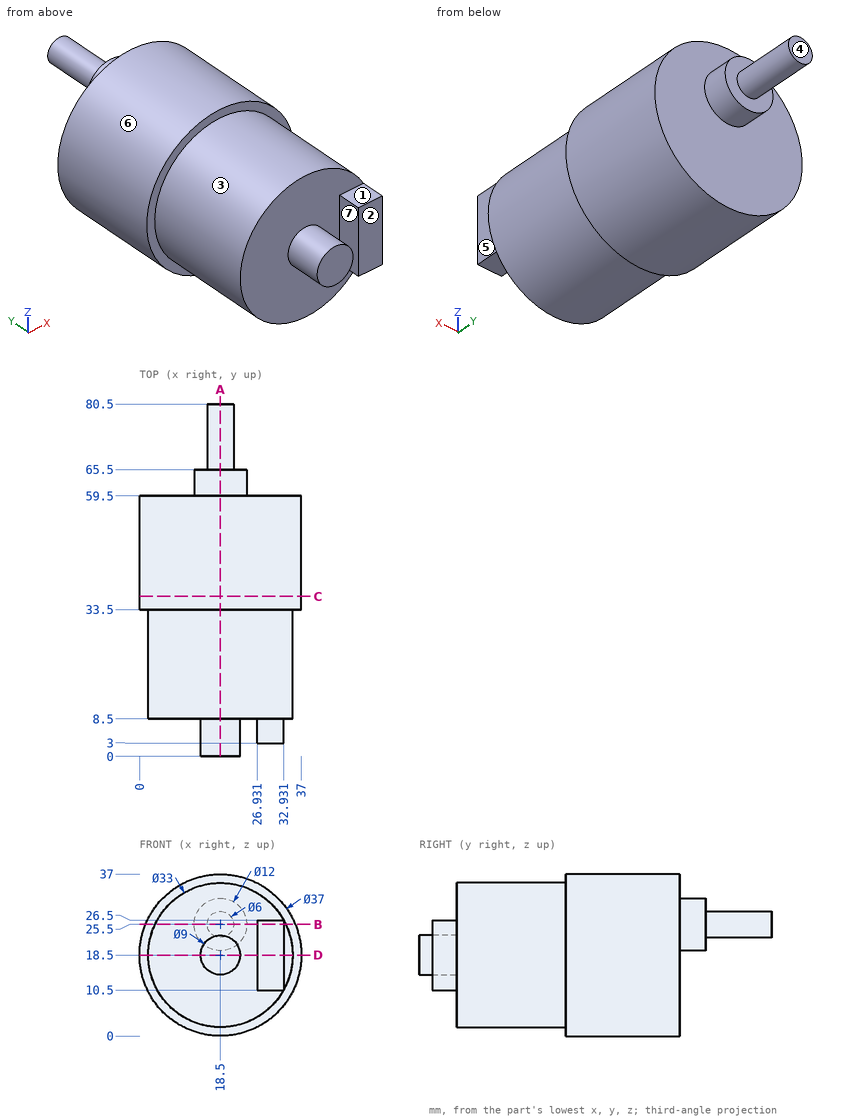
Answer from the drawing. Dimensions are ordinates in mm from the lowest x, y and z of the part. A direction names the side the tool comes from. Give positions to 0.01 mm unless a question says otherwise; leave off trailing zeros. Loops run counter-clockwise (first coordinate to the right, second up) from the corner with the lowest first, then second, coordinate; pieces in that order, holes last. Notation, with made-up numbers: (-32, -12) - (-13, -12) arc R16 ccw to (-13, 9) - close; hole circle Ø2 at (54, 81). An arc over 180 degrees is marked (long way). Write each question's results on one line, items separated by ' | '.
1. Find section D-D, the plane z = 18.5. Write down the section's boundary in (x, y), then the cut area to 3 significant figures.
Resolved:
outline: (0, 33.5) - (2, 33.5) - (2, 8.5) - (14, 8.5) - (14, 0) - (23, 0) - (23, 8.5) - (26.93, 8.5) - (26.93, 3) - (32.93, 3) - (32.93, 8.5) - (35, 8.5) - (35, 33.5) - (37, 33.5) - (37, 59.5) - (0, 59.5) - close | area: 1,900 mm^2
2. For a pull along X with two mould halves and no side action, classify the marked faces 4, 5, 6 and 7 as +X half, -X half, draft (parallel to the pull), parting line (faces both ways), or undercut.
Resolved:
face 4: draft | face 5: +X half | face 6: parting line | face 7: undercut
3. Flat-ended cylindrical pins translate along their axes: P1, Ø6, axis at y = 6.5, z = 15, coming from the +X side; P2, Ø6, axis at x = 28.5, z = 16, coming from the +Y side; P3, Ø5, axis at y = 56.5, z = 17, coming from the +X side. Find the tip coordinate at first contact, or state that the pin passes through.
Resolved:
P1: stops at x = 34.95 | P2: stops at y = 59.5 | P3: stops at x = 37
4. Find section C-C, the plane y = 36.5. Write down the section's boundary in (x, z), then the cut area to 3 significant figures.
Resolved:
outline: circle Ø37 at (18.5, 18.5) | area: 1,080 mm^2
5. Consider probe 1 along Y at (x, z) = (16.5, 29.5); probe 2 along Y at (x, z) = (11, 9.5); probe 3 along Z at (x, y) = (30, 4). Determine where each line is inside the solid, lowest interval first. Write a range as from..to.
Resolved:
probe 1: y = 8.5..65.5 | probe 2: y = 8.5..59.5 | probe 3: z = 10.5..26.5
6. Which of the six approach directions +Z, -Z, +X, -X, +Y, -Y give full straight-line access (tool end or side, diameter ignored) to the marked faces 1, 2 and 3?
Resolved:
face 1: +Z, +X, -X, -Y | face 2: +Z, -Z, +X, -Y | face 3: -Y
7. Find section B-B, the plane z = 25.5. Write down the section's boundary in (x, y), then the cut area to 3 significant figures.
Resolved:
outline: (1.38, 33.5) - (3.56, 33.5) - (3.56, 8.5) - (26.93, 8.5) - (26.93, 3) - (32.93, 3) - (32.93, 8.5) - (33.44, 8.5) - (33.44, 33.5) - (35.62, 33.5) - (35.62, 59.5) - (24.5, 59.5) - (24.5, 65.5) - (21.5, 65.5) - (21.5, 80.5) - (15.5, 80.5) - (15.5, 65.5) - (12.5, 65.5) - (12.5, 59.5) - (1.38, 59.5) - close | area: 1,830 mm^2
8. Find section A-A, the plane x = 18.5. Write down the section's boundary in (y, z), then the cut area to 3 significant figures.
Resolved:
outline: (0, 14) - (8.5, 14) - (8.5, 2) - (33.5, 2) - (33.5, 0) - (59.5, 0) - (59.5, 19.5) - (65.5, 19.5) - (65.5, 22.5) - (80.5, 22.5) - (80.5, 28.5) - (65.5, 28.5) - (65.5, 31.5) - (59.5, 31.5) - (59.5, 37) - (33.5, 37) - (33.5, 35) - (8.5, 35) - (8.5, 23) - (0, 23) - close | area: 2,030 mm^2
